from build123d import *

# Parameters (mm, degrees)
F0_R     = 12.5
F0_R_2   = 6.1
F1_DEPTH = 6
F2_DEPTH = 2
F4_DEPTH = 2.5


with BuildPart() as f1:
    # F0 (on Top) → F1 (new body)
    with BuildSketch(Plane.XY):
        Circle(F0_R)
        Circle(F0_R_2, mode=Mode.SUBTRACT)
    extrude(amount=-F1_DEPTH)

    # F0 (on Top) → F2 (join)
    with BuildSketch(Plane.XY):
        Circle(F0_R_2)
    extrude(amount=-F2_DEPTH)

    # F3 (on Front) → F4 (join, symmetric)
    with BuildSketch(Plane.XZ):
        with BuildLine():
            add(Edge.make_bspline(
                [(8.745821, 5.343975), (8.750764, 5.447785), (8.745821, 5.551827)],
                knots=[0, 0, 0, 0.067901, 0.067901, 0.067901], degree=2, weights=[1, 0.999424, 1]))
            Line((8.745821, 5.551827), (8.745821, 5.343975))
        make_face()
        with BuildLine():
            add(Edge.make_bspline(
                [(-3.056437, 1.444817), (-3.056437, 3.232295), (-5.297712, 4.106672)],
                knots=[0, 0, 0, 1.059661, 1.059661, 1.059661], degree=2, weights=[1, 0.862893, 1]))
            add(Edge.make_bspline(
                [(-5.297712, 4.106672), (-19.40331, 9.609614), (-11.229873, -0.097585), (-3.056437, -9.804784), (-3.056437, 1.444817)],
                knots=[1.059661, 1.059661, 1.059661, 3.671423, 3.671423, 6.283185, 6.283185, 6.283185], degree=2, weights=[1, 0.261827, 1, 0.261827, 1]))
        make_face()
        with BuildLine():
            Line((8.745821, 5.343975), (8.745821, 5.551827))
            add(Edge.make_bspline(
                [(8.745821, 5.551827), (8.669129, 7.165933), (6.763276, 8.076893)],
                knots=[0.067901, 0.067901, 0.067901, 1.037788, 1.037788, 1.037788], degree=2, weights=[1, 0.884701, 1]))
            add(Edge.make_bspline(
                [(6.763276, 8.076893), (2.438907, 10.143854), (0.493255, 6.802759), (-1.452398, 3.461665), (3.559705, 2.575689), (8.571808, 1.689712), (8.745821, 5.343975)],
                knots=[1.037788, 1.037788, 1.037788, 2.786254, 2.786254, 4.53472, 4.53472, 6.283185, 6.283185, 6.283185], degree=2, weights=[1, 0.641585, 1, 0.641585, 1, 0.641585, 1]))
        make_face()
        with BuildLine():
            Line((8.745821, 22.28014), (-5.297712, 19.104175))
            Line((-5.297712, 19.104175), (-5.297712, 4.106672))
            add(Edge.make_bspline(
                [(-3.056437, 1.444817), (-3.056437, 3.232295), (-5.297712, 4.106672)],
                knots=[0, 0, 0, 1.059661, 1.059661, 1.059661], degree=2, weights=[1, 0.862893, 1]))
            Line((-3.056437, 1.444817), (-3.056437, 15.368507))
            Line((-3.056437, 15.368507), (6.763276, 17.666737))
            Line((6.763276, 17.666737), (6.763276, 8.076893))
            add(Edge.make_bspline(
                [(8.745821, 5.551827), (8.669129, 7.165933), (6.763276, 8.076893)],
                knots=[0.067901, 0.067901, 0.067901, 1.037788, 1.037788, 1.037788], degree=2, weights=[1, 0.884701, 1]))
            Line((8.745821, 5.551827), (8.745821, 22.28014))
        make_face()
    extrude(amount=F4_DEPTH, both=True)


solid = f1.part
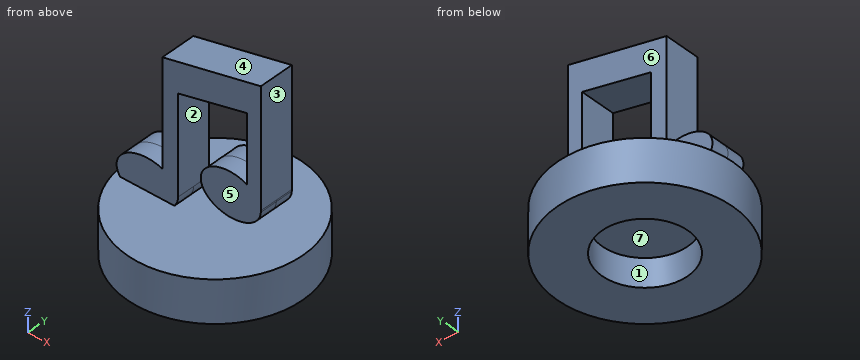
Part model, mm, in its own coordinate system. Face numbers are marked on the shaded views. A direction names the side the tool comes from. Give positions to 0.01 mm unless a question says otherwise; leave off trailing zeros. Loops run counter-clockwise (first coordinate to the right, second up) from the corner with the lowest first, then second, coordinate; pieces in that order, holes last. Notation, with made-up numbers: (-6.75, 33) -> (8.25, 33) arc R21 cw to (8.25, 58) -> close; hole circle Ø8 at (23.25, 70.5). An arc over 180 degrees is marked (long way). Write each question's results on one line, items separated by ' | '. Start each with the question number.
Q1. Band-saw the part on C-C on y = 4.5. List the corners of the cut face in (x, z).
Q2. Which spindle directions (+Z, -Z, +X, -X, +Y, -Y) get a long thin tool onto all of the face, cutting with end or side? Do the marked faces 1, 2 and 3. Say none if no direction does.
Q3. Band-saw the part on B-B on x = -2.25. List the corners of the cut face in (y, z).
Q4. Pin check, flat tips, straight feed: P1, Ø7.5, axis at x = 2, y = 4, coming from the +Z side; P2, Ø5, axis at x = 8, z = 3, coming from the +Y side; P3, Ø4, axis at y = 0.5, z = 13, coming from the -X side; P4, Ø3, axis at x = -8.5, z = 16.5, coming from the -Y side. Stop position of each tip, or through.
Q5. Band-saw the part on D-D on x = 5. Count the separate pieces of the cut face and the enclosed holes in it, plus the area to 3 significant figures.
Q6. Wall check: L1, parallel to Y at x = 0, z = -3.7; L2, parallel to Z at x = 3, y = 1.75; L3, parallel to Z at x = 2.75, y = 10.5. Give the ranges that are in metal, low to high.
Q7. Pull direction Y, two halves, no side cores. Call the marked faces 4, 5, 6 and 7: +Y half, -Y half, draft (parallel to the pull), parting line (faces both ways), or undercut.
Q8. Band-saw the part on A-A on z = 12.25. List the corners of the cut face in (x, y), plus the area to 3 significant figures.
Results are:
1) outline: (-11.66, -6) -> (-4.12, -6) -> (-4.12, -2) -> (4.12, -2) -> (4.12, -6) -> (11.66, -6) -> (11.66, 0) -> (-11.66, 0) -> close
2) face 1: -Z | face 2: +Y, -Y | face 3: +Z, +X, +Y, -Y
3) outline: (-12.3, -6) -> (-5.67, -6) -> (-5.67, -2) -> (5.67, -2) -> (5.67, -6) -> (12.3, -6) -> (12.3, 0) -> (-12.3, 0) -> close; (-2.5, 15.56) -> (2.5, 15.56) -> (2.5, 19.79) -> (-2.5, 19.79) -> close
4) P1: stops at z = 21.53 | P2: stops at y = 2.5 | P3: stops at x = -5.3 | P4: passes through
5) separate pieces: 3 | enclosed holes: 0 | area: 161 mm²
6) L1: y = -12.5 to -6.1, 6.1 to 12.5 | L2: z = -2 to 0, 2.7 to 8.46, 16.79 to 20.98 | L3: z = -6 to 0
7) face 4: draft | face 5: -Y half | face 6: +Y half | face 7: undercut
8) outline: (-5.3, -2.5) -> (-3.06, -2.5) -> (-3.06, 2.5) -> (-5.3, 2.5) -> close; (6.76, -2.5) -> (8.75, -2.5) -> (8.75, 2.5) -> (6.76, 2.5) -> close | area: 21.1 mm²
